Autodesk Inventor part; units mm, degrees
ref_plane "YZ Plane" through (0, 0, 0) normal (1, 0, 0) x (0, 1, 0)
ref_plane "XZ Plane" through (0, 0, 0) normal (0, 1, 0) x (-1, 0, 0)
ref_plane "XY Plane" through (0, 0, 0) normal (0, 0, 1) x (1, 0, 0)
sketch "Sketch1" plane through (0, 0, 0) normal (0, 0, 1) x (1, 0, 0)
  circle A0 centre (0, -7.5) radius 2.8
  line L0 (-2.2805, 10.95) -> (2.2805, 10.95)
  line L1 (2.2805, 10.95) -> (4.5611, 7)
  line L2 (4.5611, 7) -> (2.2805, 3.05)
  line L3 (2.2805, 3.05) -> (-2.2805, 3.05)
  line L4 (-2.2805, 3.05) -> (-4.5611, 7)
  line L5 (-4.5611, 7) -> (-2.2805, 10.95)
  line L6 (8.5, 13) -> (-8.5, 13)
  line L7 (-8.5, 13) -> (-8.5, -13)
  line L8 (-8.5, -13) -> (8.5, -13)
  line L9 (8.5, -13) -> (8.5, 13)
  point P0 (0, 0)
extrude "Extrusion1" add sketch "Sketch1" along normal blind 2
sketch "Sketch2" plane through (0, 0, 2) normal (0, 0, 1) x (1, 0, 0)
  line L0 (8.5, -13) -> (8.5, 13)
  line L1 (8.5, 13) -> (-8.5, 13)
  line L2 (-8.5, 13) -> (-8.5, -13)
  line L3 (-8.5, -13) -> (8.5, -13)
  point P0 (0, 0)
extrude "Extrusion2" add sketch "Sketch2" along normal blind 2
sketch "Sketch3" plane through (-8.5, 13, 0) normal (0, 1, 0) x (1, 0, 0)
  circle A0 centre (8.5, -8.75) radius 2.75
  circle A1 centre (8.5, -8.75) radius 1.05
  line L0 (0, -4) -> (17, -4) construction
  line L1 (8.5, -4) -> (8.5, -22.1376) construction
  point P0 (8.5, 0)
  dimension "d4" = 5.5
  dimension "d5" = 2.1
  dimension "d6" = 4.75
extrude "Extrusion3" add sketch "Sketch3" along normal blind 10
sketch "Sketch4" plane through (0, 13, 8.75) normal (0, -1, 0) x (1, 0, 0)
  circle A0 centre (0, 0) radius 2.75
  line L0 (-2.75, 0) -> (2.75, 0)
  line L1 (2.75, 0) -> (2.75, -4.75)
  line L2 (2.75, -4.75) -> (-2.75, -4.75)
  line L3 (-2.75, -4.75) -> (-2.75, 0)
  line L4 (-8.5, -4.75) -> (8.5, -4.75)
  point P0 (0, -8.75)
extrude "Extrusion4" add sketch "Sketch4" along normal up to surface (26 mm away)
properties part number "connector9V"
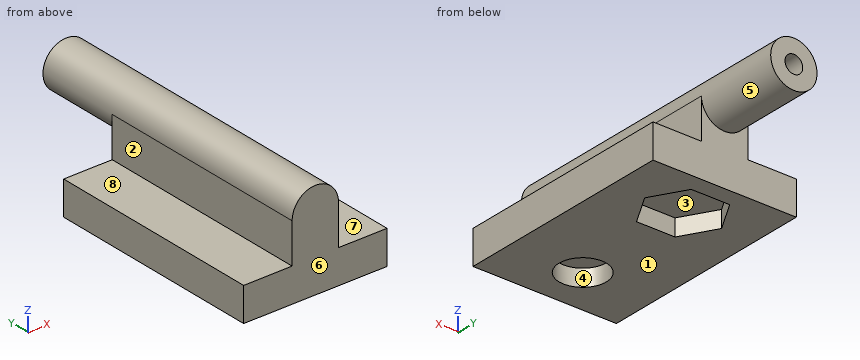
Input: part model. Units: mm. Frame: model coordinates. Face numbers are marked on the shaded views. A direction names the side the tool comes from. Give positions to 0.01 mm unless a question says otherwise; leave off trailing zeros. Order: outer loops, then holes, each group sorted by start corner. A loop starts at its lowest first (then second) coordinate and runs counter-clockwise, first axis right, second up. Notation, with made-up numbers: (-33, -26.75) - (-6, -26.75) arc R23 ccw to (-6, -17.75) - close; hole circle Ø3 at (55.5, 14.5). An arc over 180 degrees is marked (long way). Use a Markdown table: item, result.
(1) Draft query along X for the marked faces 1, 2 and 3. Return one class per face: released by +X, released by -X, zero draft, split by the parting line, or undercut.
Computed values:
| item | result |
|---|---|
| face 1 | zero draft |
| face 2 | released by -X |
| face 3 | undercut |
(2) Section query A-A (x = 0). Output: boundary loops of the cut face in (y, z).
Computed values:
| item | result |
|---|---|
| outline | (-13, 0) - (-10.3, 0) - (-10.3, 2) - (-4.7, 2) - (-4.7, 0) - (3.05, 0) - (3.05, 2) - (10.95, 2) - (10.95, 0) - (13, 0) - (13, 6) - (23, 6) - (23, 7.7) - (13, 7.7) - (13, 9.8) - (23, 9.8) - (23, 11.5) - (-13, 11.5) - close |
(3) Section query B-B (y = -7.5). Output: boundary loops of the cut face in (x, z).
Computed values:
| item | result |
|---|---|
| outline | (-8.5, 0) - (-2.8, 0) - (-2.8, 2) - (2.8, 2) - (2.8, 0) - (8.5, 0) - (8.5, 4) - (2.75, 4) - (2.75, 8.75) arc R2.75 ccw to (-2.75, 8.75) - (-2.75, 4) - (-8.5, 4) - close |
(4) Line query: line 1 (Y direction, x = 0, z = 1.1); line 2 (X direction, y = 16, z = 8.75); line 3 (Z direction, x = 3.5, y = -7). Output: solid intervals per line, ascending. Write a range as from..to.
Computed values:
| item | result |
|---|---|
| line 1 | y = -13..-10.3, -4.7..3.05, 10.95..13 |
| line 2 | x = -2.75..-1.05, 1.05..2.75 |
| line 3 | z = 0..4 |
(5) Section query C-C (z = 5.25). Output: boundary loops of the cut face in (x, y).
Computed values:
| item | result |
|---|---|
| outline | (-2.75, -13) - (2.75, -13) - (2.75, 13) - (-2.75, 13) - close |
(6) Section query D-D (y = -3). Output: boundary loops of the cut face in (x, z), then the cut area to 3 significant figures.
Computed values:
| item | result |
|---|---|
| outline | (-8.5, 0) - (8.5, 0) - (8.5, 4) - (2.75, 4) - (2.75, 8.75) arc R2.75 ccw to (-2.75, 8.75) - (-2.75, 4) - (-8.5, 4) - close |
| area | 106 mm2 |
(7) Access query for the marked faces 4, 5, 6, 7 and 8. Directions: +Z, -Z, +X, -X, +Y, -Y. A direction counts if a zero-diameter tool reaches every point of the face in a straight line with its end or side. Return the directions, or none.
Computed values:
| item | result |
|---|---|
| face 4 | -Z |
| face 5 | +Y |
| face 6 | +Z, -Z, +X, -X, -Y |
| face 7 | +Z, +X, +Y, -Y |
| face 8 | +Z, -X, +Y, -Y |
(8) Pin query (flat end, axial travel): pin 1 (5 mm diameter, centred on y = 12.5, z = 9, fed in from -X); pin 2 (4 mm diameter, centred on y = -4, z = 7, fed in from +X); pin 3 (1.7 mm diameter, centred on x = -0.5, z = 9, fed in from +Y); pin 4 (1 mm diameter, centred on x = -1.5, z = 3, fed in from +Y). Return the tip coordinate at first contact, or that it passes through.
Computed values:
| item | result |
|---|---|
| pin 1 | stops at x = -2.75 |
| pin 2 | stops at x = 2.75 |
| pin 3 | stops at y = 23 |
| pin 4 | stops at y = 13 |
